Check sheet for the modelled part. Datum: model origin and axes. Units: mm. A direction names the side the tool comes from. Round coordinates to 2 decimals unless told otherwise and drop trailing zeros. Write each loop counter-clockwise with the first axis right and the second up, starting at its lowest first coordinate (ties: lowest second). Pieces come first, ordered by that corner, then holes. Notation, with made-up numbers: (74, 34) - (109, 34) arc R33 ccw to (109, 69) - close; hole circle Ø2 at (-35.75, 59.25). An arc over 180 degrees is marked (long way). Use one line per item in the form item = value. Start each with the question number.
1) Scan lines: probe 1 along X at (y, z) = (-0.1, 3.5); probe 2 along X at (y, z) = (-1.2, 0.25); probe 3 along Z at (x, y) = (0.25, 0.35). Record each from-to range of solid material in increasing order.
2) Section check C-C (y = -0.75). Record the boundary of the cut face in (x, z), then the cut area to 3 significant figures.
3) Set-up check for faces 4 (the face through (0, 0, -4.5)), 5 (the face through (-3.07, 1.05, 0.06)): record each of +Z, -Z, +X, -X, +Y, -Y from which the full face is reachable in a straight line by a thin tool's end or side.
4) Gauge pin test, flat ends, axial feed: P1, Ø0.8, axis at x = 0, y = -0.5, coming from the -Z side; P2, Ø1, axis at y = -1, z = -1.5, coming from the +X side; P3, Ø1.2, axis at y = 0.5, z = 2, coming from the +X side; P4, Ø0.8, axis at y = -0.5, z = 0.5, coming from the -X side. Record the tip position at first contact, or that the pin passes through.
5) Draft check along X on faces 1 (the face through (3.05, -1.07, -0.06)), 2 (the face through (1.7, -1.5, -0.1)), 3 (the face through (0, 0, 4.5)). Enter one of: +X half, -X half, draft (parallel to the pull), parting line (faces both ways), or undercut.
from build123d import *

# Parameters (mm, degrees)
SKETCH1_W      = 7
SKETCH1_H      = 16
SKETCH1_W_2    = 2
SKETCH1_H_2    = 9
EXTRUDE1_DEPTH = 1.5
FILLET1_RADIUS = 3.5
FILLET1_LENGTH = 3
FILLET5_RADIUS = 3.5
FILLET5_LENGTH = 3
FILLET3_R      = 0.25
FILLET4_R      = 0.25
FILLET6_R      = 1.5


with BuildPart() as part:
    # Sketch1 → Extrude1 (new, symmetric)
    with BuildSketch(Plane(origin=(0, 0, 0), x_dir=(1, 0, 0), z_dir=(0, 1, 0))):
        Rectangle(SKETCH1_W, SKETCH1_H)
        Rectangle(SKETCH1_W_2, SKETCH1_H_2, mode=Mode.SUBTRACT)
    extrude(amount=EXTRUDE1_DEPTH, both=True)

    # Fillet1: full round fillet: the end face becomes a half cylinder, R = half its width
    fillet1_face = Plane((0, 0, 8), x_dir=(0, 1, 0), z_dir=(0, 0, 1))  # on the end face: x along it, z out of the body
    fillet1_slab = fillet1_face.offset(-FILLET1_RADIUS / 2) * Box(FILLET1_LENGTH, 2 * FILLET1_RADIUS, FILLET1_RADIUS, mode=Mode.PRIVATE)  # the body's end, R deep
    fillet1_round = Plane((0, 0, 4.5), x_dir=(0, 0, 1), z_dir=(0, 1, 0)) * Cylinder(FILLET1_RADIUS, FILLET1_LENGTH, mode=Mode.PRIVATE)  # its axis R under the face
    add(fillet1_slab - fillet1_round, mode=Mode.SUBTRACT)

    # Fillet5: full round fillet: the end face becomes a half cylinder, R = half its width
    fillet5_face = Plane((0, 0, -8), x_dir=(0, 1, 0), z_dir=(0, 0, -1))  # on the end face: x along it, z out of the body
    fillet5_slab = fillet5_face.offset(-FILLET5_RADIUS / 2) * Box(FILLET5_LENGTH, 2 * FILLET5_RADIUS, FILLET5_RADIUS, mode=Mode.PRIVATE)  # the body's end, R deep
    fillet5_round = Plane((0, 0, -4.5), x_dir=(0, 0, -1), z_dir=(0, 1, 0)) * Cylinder(FILLET5_RADIUS, FILLET5_LENGTH, mode=Mode.PRIVATE)  # its axis R under the face
    add(fillet5_slab - fillet5_round, mode=Mode.SUBTRACT)

    # Fillet3
    fillet3_edges = [part.edges().sort_by_distance(p)[0] for p in [
        (-1, 0, -4.5),
        (-1, 0, 4.5),
        (1, 0, 4.5),
        (1, 0, -4.5),
    ]]
    fillet(fillet3_edges, radius=FILLET3_R)

    # Fillet4
    fillet4_edges = [part.edges().sort_by_distance(p)[0] for p in [
        (1, -1.5, 0),
        (1, 1.5, 0),
        (0, -1.5, -4.5),
        (0, 1.5, -4.5),
        (-1, -1.5, 0),
        (-1, 1.5, 0),
        (0, -1.5, 4.5),
        (0, 1.5, 4.5),
        (0.926776695, -1.5, -4.426776695),
        (0.926776695, 1.5, -4.426776695),
        (-0.926776695, -1.5, -4.426776695),
        (-0.926776695, 1.5, -4.426776695),
        (0.926776695, -1.5, 4.426776695),
        (0.926776695, 1.5, 4.426776695),
        (-0.926776695, -1.5, 4.426776695),
        (-0.926776695, 1.5, 4.426776695),
    ]]
    fillet(fillet4_edges, radius=FILLET4_R)

    # Fillet6
    fillet6_edges = [part.edges().sort_by_distance(p)[0] for p in [
        (3.5, -1.5, 0),
        (3.5, 1.5, 0),
        (0, 1.5, 8),
        (-3.5, -1.5, 0),
        (-3.5, 1.5, 0),
        (0, -1.5, -8),
    ]]
    fillet(fillet6_edges, radius=FILLET6_R - 0.0001)  # a hair under: the kernel refuses the full size


solid = part.part
Results are:
q1.probe_1 = -3.5 to -1, 1 to 3.5
q1.probe_2 = -2.9 to -1, 1 to 2.9
q1.probe_3 = -7.95 to -4.5, 4.5 to 7.95
q2.outline = (-3.3, -4.5) arc R3.3 ccw to (3.3, -4.5) - (3.3, 4.5) arc R3.3 ccw to (-3.3, 4.5) - close; hole (-1, -4.25) arc R0.25 ccw to (-0.75, -4.5) - (0.75, -4.5) arc R0.25 ccw to (1, -4.25) - (1, 4.25) arc R0.25 ccw to (0.75, 4.5) - (-0.75, 4.5) arc R0.25 ccw to (-1, 4.25) - close
q2.area = 75.6 mm²
q3.face_4 = +Y, -Y
q3.face_5 = +Z, -Z, -X, +Y
q4.P1 = -8
q4.P2 = 3.41
q4.P3 = 3.5
q4.P4 = -3.5
q5.face_1 = +X half
q5.face_2 = draft
q5.face_3 = undercut
